Could you check a few things on this model? Use its own coordinates, in mm. Face numbers are marked on the shaded views. A direction names the side the tool comes from. Round coordinates to 2 decimals unless told otherwise and drop trailing zeros. Order: outer loops, then holes, each group sorted by start corner. A loop starts at its lowest first (then second) coordinate and runs counter-clockwise, first axis right, second up. Notation, with made-up numbers: (53, 24.5) -> (73, 24.5) arc R6 ccw to (73, 35.5) -> close; hole circle Ø2 at (-29.75, -19). An arc over 180 degrees is marked (long way). One line per question, with ' | ' between items.
```python
from build123d import *

# Parameters (mm, degrees)
SKETCH1_W           = 17
SKETCH1_H           = 17
BOSS_EXTRUDE1_DEPTH = 4
SKETCH2_W           = 14
SKETCH2_H           = 14
CUT_EXTRUDE1_DEPTH  = 2.5
FILLET1_R           = 2
FILLET2_R           = 3.5
SKETCH3_W           = 2.5
SKETCH3_H           = 1.5
CUT_EXTRUDE2_DEPTH  = 1.5
FILLET3_R           = 2


with BuildPart() as part:
    # Sketch1 → Boss-Extrude1 (new body)
    with BuildSketch(Plane.XY):
        with Locations((8.5, 8.5)):
            Rectangle(SKETCH1_W, SKETCH1_H)
    extrude(amount=BOSS_EXTRUDE1_DEPTH)

    # Sketch2 → Cut-Extrude1 (cut)
    with BuildSketch(Plane.XY.offset(4)):
        with Locations((8.5, 8.5)):
            Rectangle(SKETCH2_W, SKETCH2_H)
    extrude(amount=-CUT_EXTRUDE1_DEPTH, mode=Mode.SUBTRACT)

    # Fillet1
    fillet1_edges = [part.edges().sort_by_distance(p)[0] for p in [
        (1.5, 1.5, 2.75),
        (1.5, 15.5, 2.75),
        (15.5, 15.5, 2.75),
        (15.5, 1.5, 2.75),
    ]]
    fillet(fillet1_edges, radius=FILLET1_R)

    # Fillet2
    fillet2_edges = [part.edges().sort_by_distance(p)[0] for p in [
        (0, 17, 2),
        (17, 17, 2),
        (17, 0, 2),
        (0, 0, 2),
    ]]
    fillet(fillet2_edges, radius=FILLET2_R)

    # Sketch3 → Cut-Extrude2 (cut)
    with BuildSketch(Plane.XY.offset(4)):
        with Locations((4.75, 0.75)):
            Rectangle(SKETCH3_W, SKETCH3_H)
    extrude(amount=-CUT_EXTRUDE2_DEPTH, mode=Mode.SUBTRACT)

    # Fillet3
    fillet3_edges = [part.edges().sort_by_distance(p)[0] for p in [
        (17, 8.5, 0),
        (0, 8.5, 0),
        (8.5, 17, 0),
        (8.5, 0, 0),
        (1.025126266, 15.974873734, 0),
        (15.974873734, 15.974873734, 0),
        (1.025126266, 1.025126266, 0),
        (15.974873734, 1.025126266, 0),
    ]]
    fillet(fillet3_edges, radius=FILLET3_R)


solid = part.part
```
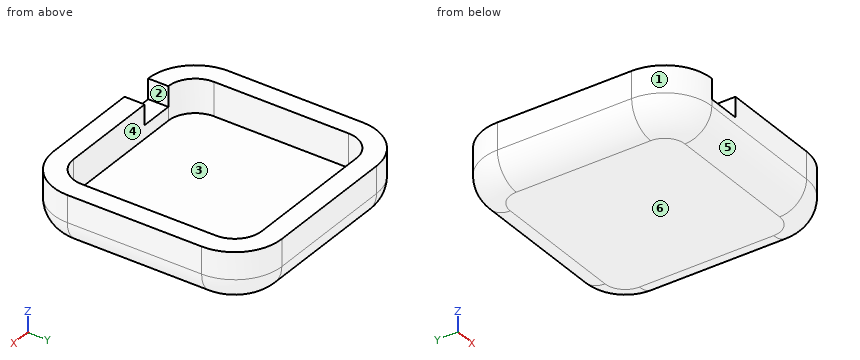
1. I want a section at C-C on z = 2.95. List the corners of the cut face in (x, y) for me.
From the geometry:
outline: (0, 3.5) arc R3.5 ccw to (3.5, 0) -> (3.5, 1.5) arc R2 cw to (1.5, 3.5) -> (1.5, 13.5) arc R2 cw to (3.5, 15.5) -> (13.5, 15.5) arc R2 cw to (15.5, 13.5) -> (15.5, 3.5) arc R2 cw to (13.5, 1.5) -> (6, 1.5) -> (6, 0) -> (13.5, 0) arc R3.5 ccw to (17, 3.5) -> (17, 13.5) arc R3.5 ccw to (13.5, 17) -> (3.5, 17) arc R3.5 ccw to (0, 13.5) -> close
2. If we mould it in two halves opening along Y, with no side actions, what happens to the marked faces 4, 5 and 6? For each: pulls with the +Y half, pulls with the -Y half, needs draft (parallel to the pull), parting line crosses it, or undercut.
From the geometry:
face 4: undercut | face 5: pulls with the -Y half | face 6: needs draft
3. I'm going to push flat-ended pins straight in: pin 1 (0.8 mm diameter, centred on y = 0.5, z = 3.5, fed in from -X); pin 2 (5 mm diameter, centred on x = 4.5, y = 6.5, fed in from +Z); pin 3 (10 mm diameter, centred on x = 13.5, y = 11.5, fed in from +Z); pin 4 (1.6 mm diameter, centred on y = 0.5, z = 3, fed in from +X). Where does each tip first touch, or does it pass through?
From the geometry:
pin 1: stops at x = 1.16 | pin 2: stops at z = 1.5 | pin 3: stops at z = 4 | pin 4: stops at x = 16.22
4. I want a section at A-A on x = 8.5. List the corners of the cut face in (y, z) for me, and give its area (3 significant figures).
From the geometry:
outline: (0, 2) arc R2 ccw to (2, 0) -> (15, 0) arc R2 ccw to (17, 2) -> (17, 4) -> (15.5, 4) -> (15.5, 1.5) -> (1.5, 1.5) -> (1.5, 4) -> (0, 4) -> close | area: 31.3 mm²
5. On a 3-axis mill with a long thin cutter (end or side, diameter ignored), from which of +Z, -Z, +X, -X, +Y, -Y can I reach the whole of each face in a straight line? I mean the marked faces 1, 2 and 3. Say none if no direction works.
From the geometry:
face 1: +Z, -Z, -X, -Y | face 2: +Z, -Y | face 3: +Z
6. I need wall thicknesses on probe 1 along Y at (x, z) = (10, 3.5); probe 2 along X at (y, z) = (2.5, 1.85). Which ranges of each line are inside material? Lowest first, please.
From the geometry:
probe 1: y = 0 to 1.5, 15.5 to 17 | probe 2: x = 0.15 to 1.77, 15.23 to 16.85
